```python
from build123d import *

# Parameters (mm, degrees)
BOSS_EXTRUDE1_DEPTH        = 2.54
F_7_0_201_DIAMETER_HOLE1_D = 5.1054
FILLET1_R                  = 3.175


with BuildPart() as part:
    # Sketch1 → Boss-Extrude1 (new body)
    with BuildSketch(Plane(origin=(0, 0, 0), x_dir=(1, 0, 0), z_dir=(0, 1, 0))):
        Polygon((0, 0), (-38.15203444, 103.451714303), (-29.4647228, 127.319906871), (89.87624004, 83.883348669), (81.1889284, 60.015156101), (25.4, 0), align=None)
    extrude(amount=BOSS_EXTRUDE1_DEPTH)

    # #7 (0.201) Diameter Hole1 (through all)
    with Locations(Plane(origin=(0, 0, 0), x_dir=(-1, 0, 0), z_dir=(0, -1, 0))):
        with Locations((-73.598487936, 76.292908205), (-49.730295368, 84.980219846), (-25.8621028, 93.667531486), (-1.993910232, 102.354843126), (21.874282336, 111.042154767), (-12.7, 63.5), (-12.7, 38.1), (-12.7, 12.7)):
            Hole(F_7_0_201_DIAMETER_HOLE1_D / 2)

    # Fillet1
    fillet1_edges = [part.edges().sort_by_distance(p)[0] for p in [
        (0, 1.27, 0),
        (-38.15203444, 1.27, -103.451714303),
        (-29.4647228, 1.27, -127.319906871),
        (89.87624004, 1.27, -83.883348669),
        (81.1889284, 1.27, -60.015156101),
        (25.4, 1.27, 0),
    ]]
    fillet(fillet1_edges, radius=FILLET1_R)


solid = part.part
```
The model under review builds one solid part; all positions refer to its coordinate system, in mm. Coordinates: 2 decimals unless noted, no trailing zeros. Order: outer loops, then holes, each group sorted by start corner. A loop starts at its lowest first (then second) coordinate and runs counter-clockwise, first axis right, second up. Notation, with made-up numbers: (18.25, -28) -> (56.25, -28) arc R16 cw to (56.25, -24) -> close; hole circle Ø11 at (34.5, 33.25). An arc over 180 degrees is marked (long way). Answer in a Markdown table with one row per item. Add a question column.
Item 1: Clearance check with flat-ended pins moving along their axes: pin 1 (4 mm diameter, centred on x = 12.7, z = -38.1, fed in from +Y); pin 2 (1 mm diameter, centred on y = 0.5, z = -67.5, fed in from -X); pin 3 (1.5 mm diameter, centred on x = 16.5, y = 1, fed in from -Z). State where each tip first meets the part, or that it passes through.
Item 2: Mouldability with a two-part tool opening along X and no side actions: class faces 1 (the cylindrical face through (-22.43, 1.29, -108.55)), 2 (the flat face through (26, 0, -64)), 3 (the flat face through (29.41, 1.25, -105.89)) as +X half, -X half, draft (parallel to the pull), parting line (faces both ways), or undercut.
Item 3: We need section A-A on z = -38.1. Write out the cut boundary in (x, y), plus the area to 3 significant figures.
Item 4: We need section D-D on z = -12.7. Write out the cut boundary in (x, y).
Item 5: To check wall thickness, follow probe 1 along Z at (x, y) = (12.7, 1.2); probe 2 along Z at (x, y) = (75, 0.8); probe 3 along X at (y, z) = (1.05, -76). State the ranges of each line that lie inside material, in increasing order.
Item 6: We need section C-C on y = 1.95. Give the number of separate pieces and of enclosed holes in the cut face, plus the area to 3 significant figures.
Item 7: We need section B-B on x = 12.7. Write out the cut boundary in (y, z), plus the area to 3 significant figures.
Final values:
| question | item | result |
|---|---|---|
| 1 | pin 1 | passes through |
| 1 | pin 2 | stops at x = -25.08 |
| 1 | pin 3 | stops at z = -110.86 |
| 2 | face 1 | undercut |
| 2 | face 2 | draft |
| 2 | face 3 | +X half |
| 3 | outline | (-14.05, 0) -> (10.15, 0) -> (10.15, 2.54) -> (-14.05, 2.54) -> close; (15.25, 0) -> (60.82, 0) -> (60.82, 2.54) -> (15.25, 2.54) -> close |
| 3 | area | 177 mm2 |
| 4 | outline | (-4.68, 0) -> (10.15, 0) -> (10.15, 2.54) -> (-4.68, 2.54) -> close; (15.25, 0) -> (37.21, 0) -> (37.21, 2.54) -> (15.25, 2.54) -> close |
| 5 | probe 1 | z = -111.97 to -66.05, -60.95 to -40.65, -35.55 to -15.25, -10.15 to 0 |
| 5 | probe 2 | z = -89.3 to -78.43, -74.16 to -53.36 |
| 5 | probe 3 | x = -28.03 to 71.06, 76.13 to 87.01 |
| 6 | separate pieces | 1 |
| 6 | enclosed holes | 8 |
| 6 | area | 9,160 mm2 |
| 7 | outline | (0, -111.97) -> (2.54, -111.97) -> (2.54, -66.05) -> (0, -66.05) -> close; (0, -60.95) -> (2.54, -60.95) -> (2.54, -40.65) -> (0, -40.65) -> close; (0, -35.55) -> (2.54, -35.55) -> (2.54, -15.25) -> (0, -15.25) -> close; (0, -10.15) -> (2.54, -10.15) -> (2.54, 0) -> (0, 0) -> close |
| 7 | area | 246 mm2 |
